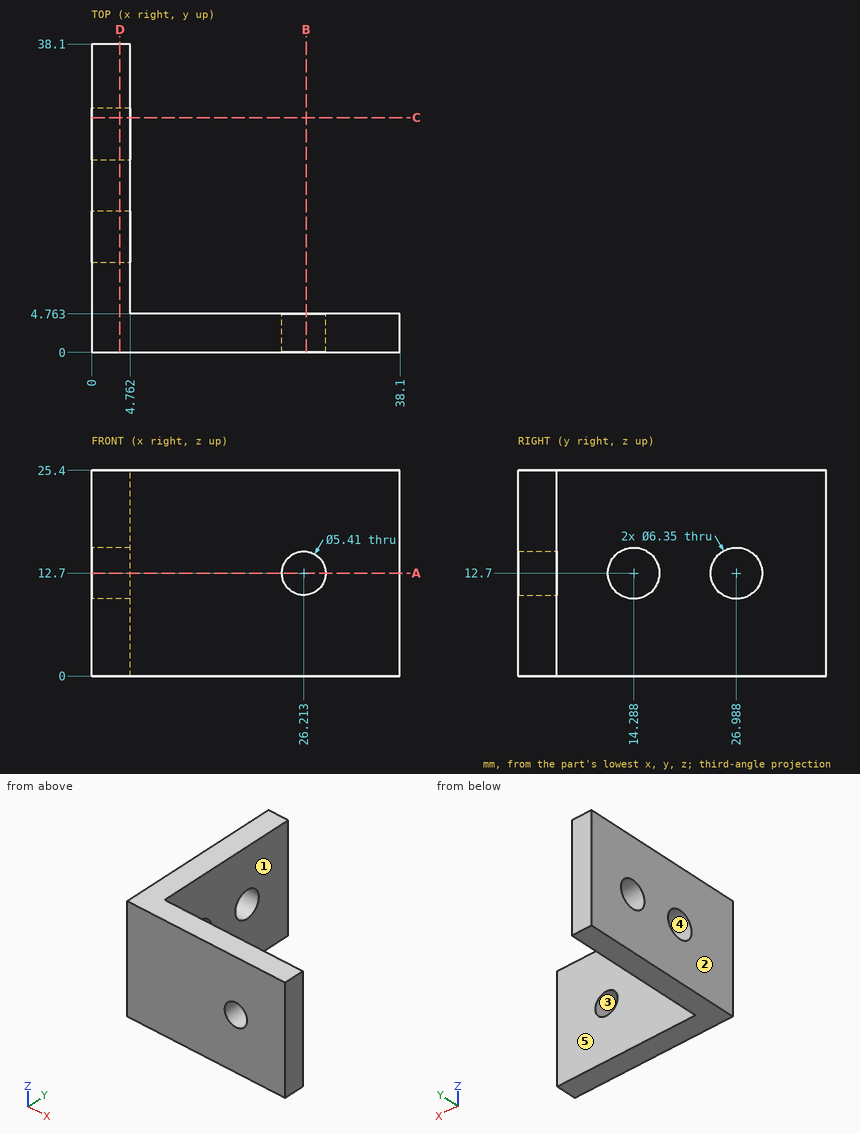
Part print with two shaded views. Sizes in mm from the minimum x, y, z corner. A direction names the side the tool comes from. Round coordinates to 2 decimals unless told otherwise and drop trailing zeros. Write each loop counter-clockwise with the first axis right and the second up, starting at its lowest first coordinate (ties: lowest second). Pieces come first, ordered by that corner, then holes. Notation, with made-up numbers: (-29.5, 52) - (7.5, 52) arc R9 ccw to (7.5, 66) - close; hole circle Ø3 at (18.25, 19.25). An arc over 180 degrees is marked (long way). Answer as CSV lines item,"result".
Q1. Tool access for the marked faces 1 and 2: list every direction of +Z, -Z, +X, -X, +Y, -Y with a clear straight run to the whole face (end or side of a thin tool).
Report:
face 1,"+Z, -Z, +X, +Y"
face 2,"+Z, -Z, -X, +Y, -Y"
Q2. Cut at C-C (y = 29). Write the cut outline in (x, z) (1 decimal).
Report:
outline,"(0, 0) - (4.8, 0) - (4.8, 10.2) - (0, 10.2) - close; (0, 15.2) - (4.8, 15.2) - (4.8, 25.4) - (0, 25.4) - close"
Q3. Drill centre lines: probe 1 along Y at (x, z) = (13.5, 13.25); probe 2 along Z at (x, y) = (4.5, 25) (1 decimal). Where is each one in solid material? Low to high. Write a range as [from, to].
Report:
probe 1,"y = [0, 4.76]"
probe 2,"z = [0, 10.2], [15.2, 25.4]"
Q4. Cut at A-A (z = 12.7). Write the cut outline in (x, y), and give its area (3 significant figures).
Report:
outline,"(0, 0) - (23.51, 0) - (23.51, 4.76) - (4.76, 4.76) - (4.76, 11.11) - (0, 11.11) - close; (0, 17.46) - (4.76, 17.46) - (4.76, 23.81) - (0, 23.81) - close; (0, 30.16) - (4.76, 30.16) - (4.76, 38.1) - (0, 38.1) - close; (28.92, 0) - (38.1, 0) - (38.1, 4.76) - (28.92, 4.76) - close"
area,"254 mm^2"
Q5. Cut at D-D (x = 3.5). State how many separate pieces and enclosed holes the cut face has.
Report:
separate pieces,"1"
enclosed holes,"2"
Q6. Cut at B-B (x = 26.5). Write the cut outline in (y, z).
Report:
outline,"(0, 0) - (4.76, 0) - (4.76, 10.01) - (0, 10.01) - close; (0, 15.39) - (4.76, 15.39) - (4.76, 25.4) - (0, 25.4) - close"
Q7. Drop flat-ended pins along their axis: pin 1 (5 mm diameter, centred on y = 14, z = 8.5, fed in from +X); pin 2 (6 mm diameter, centred on x = 23, y = 8, fed in from +Z). Give the stop position or say it passes through.
Report:
pin 1,"stops at x = 4.76"
pin 2,"passes through"
Q8. Pull direction Y, two halves, no side cores. Call the marked faces 3, 4 and 5: +Y half, -Y half, draft (parallel to the pull), parting line (faces both ways), or undercut.
Report:
face 3,"draft"
face 4,"undercut"
face 5,"+Y half"
